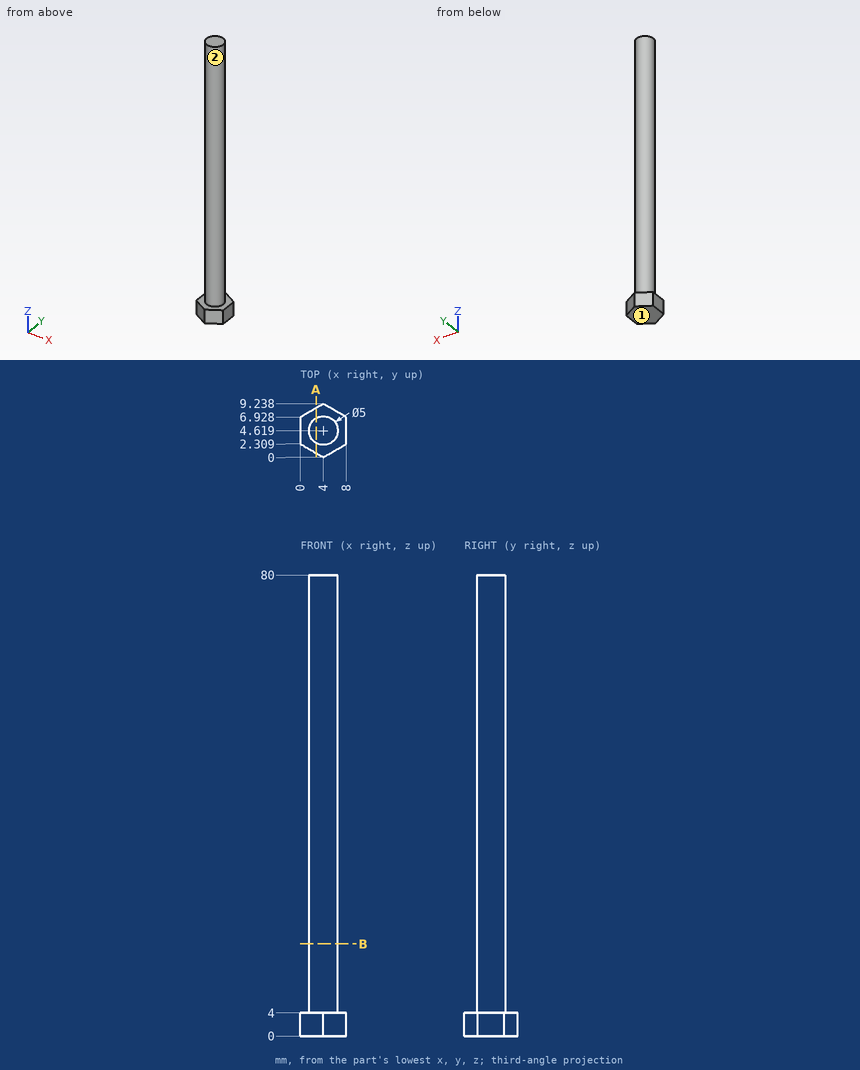
For this review, use the dimensioned drawing (mm, ordinates from the lowest corner) and the shaded views. A direction names the side the tool comes from. Coordinates: 2 decimals unless noted, no trailing zeros. Write each loop counter-clockwise with the first axis right and the second up, starting at its lowest first coordinate (ties: lowest second). Pieces come first, ordered by that corner, then holes. Notation, with made-up numbers: (-24.5, -17) - (-5.5, -17) arc R24 cw to (-5.5, 14) - close; hole circle Ø11 at (-1, -10). An arc over 180 degrees is marked (long way). Answer in a Markdown table with one row per item. Add a question column.
Q1. Clearance check with flat-ended pins moving along their axes: pin 1 (3 mm diameter, centred on x = 6.5, z = 64.5, fed in from -Y); pin 2 (4 mm diameter, centred on y = 5, z = 10.5, fed in from -X). State where each tip first meets the part, or that it passes through.
Q2. Consider section A-A on x = 2.75. Give the boundary of the cut face in (y, z), then the cut area to 3 significant figures.
Q3. To check wall thickness, follow line 1 along Z through (x, y) = (7.5, 4); line 2 along X through (y, z) = (4.5, 58.5); line 3 along Y through (x, z) = (4, 76). State the ranges of each line that lie inside material, in increasing order. Write a range as from..to.
Q4. For the marked faces 1 and 2, list the 3-axis set-ups (+Z, -Z, +X, -X, +Y, -Y) from which the entire face can be reached by the end or side of a thin tool; tool diameter is ignored.
Q5. Consider section B-B on z = 16. Give the boundary of the cut face in (x, y).
Answers below:
| question | item | result |
|---|---|---|
| 1 | pin 1 | y = 2.33 |
| 1 | pin 2 | x = 1.5 |
| 2 | outline | (0.72, 0) - (8.52, 0) - (8.52, 4) - (6.78, 4) - (6.78, 80) - (2.45, 80) - (2.45, 4) - (0.72, 4) - close |
| 2 | area | 360 mm² |
| 3 | line 1 | 0..4 |
| 3 | line 2 | 1.5..6.5 |
| 3 | line 3 | 2.12..7.12 |
| 4 | face 1 | -Z, +X, -X, +Y, -Y |
| 4 | face 2 | +Z |
| 5 | outline | circle Ø5 at (4, 4.62) |
